CAD build for the part. Positions are in the model's coordinates, mm. A direction names the side the tool comes from. Round coordinates to 2 decimals unless told otherwise and drop trailing zeros. Loops run counter-clockwise (first coordinate to the right, second up) from the corner with the lowest first, then second, coordinate; pieces in that order, holes last. Notation, with made-up numbers: (40.5, 5.5) - (90.5, 5.5) arc R10 cw to (90.5, 9.5) - close; hole circle Ø11 at (50.5, -28.5). An arc over 180 degrees is marked (long way). Use one line per item in the form item = value.
from build123d import *

# Parameters (mm, degrees)
SZKIC2_R                         = 1.65
DODANIE_WYCI_GNI_CIE1_DEPTH      = 3
DODANIE_WYCI_GNI_CIE2_DEPTH      = 5
DODANIE_WYCI_GNI_CIE3_REACH      = 30.62
DODANIE_WYCI_GNI_CIE3_START      = -1
SZKIC7_R                         = 5
SZKIC9_W                         = 12
SZKIC9_H                         = 12
DODANIE_WYCI_GNI_CIE4_DEPTH      = 16
SZKIC10_R                        = 4.1
WYTNIJ_WYCI_GNI_CIE1_DEPTH       = 18
SZKIC12_R                        = 37.17284924
WYTNIJ_WYCI_GNI_CIE2_DEPTH       = 43.690783477
SZKIC13_R                        = 3
WYTNIJ_WYCI_GNI_CIE3_DEPTH       = 42.220824259
SZKIC14_R                        = 1.65
WYTNIJ_WYCI_GNI_CIE4_DEPTH       = 42.220824259
DODANIE_WYCI_GNI_CIE5_DEPTH      = 3
DODANIE_WYCI_GNI_CIE5_DEPTH_BACK = 6
DODANIE_WYCI_GNI_CIE6_REACH      = 55.451
SZKIC16_W                        = 12
SZKIC16_H                        = 5.223766812
SZKIC17_R                        = 1.65
WYTNIJ_WYCI_GNI_CIE5_DEPTH       = 54.450515696
WYTNIJ_WYCI_GNI_CIE6_DEPTH       = 1


with BuildPart() as part:
    # Szkic2 → Dodanie-wyciągnięcie1 (new body)
    with BuildSketch(Plane(origin=(0, 0, 0), x_dir=(1, 0, 0), z_dir=(0, 1, 0))):
        with BuildLine():
            Line((4, 11), (4, -11))
            ThreePointArc((4, -11), (0, -15), (-4, -11))
            Line((-4, -11), (-4, 11))
            ThreePointArc((-4, 11), (0, 15), (4, 11))
        make_face()
        with Locations(Location((0, -11, 0), (0, 0, 270))):
            Circle(SZKIC2_R, mode=Mode.SUBTRACT)
        with Locations(Location((0, 11, 0), (0, 0, 270))):
            Circle(SZKIC2_R, mode=Mode.SUBTRACT)
    extrude(amount=DODANIE_WYCI_GNI_CIE1_DEPTH)

    # Szkic3 → Dodanie-wyciągnięcie2 (add)
    with BuildSketch(Plane(origin=(0, 3, 0), x_dir=(1, 0, 0), z_dir=(0, 1, 0))):
        Polygon((6, 16), (6, -14), (6, -20), (-6, -20), (-6, -14), (-6, 16), (-6, 22), (6, 22), align=None)
        with BuildLine():
            Line((3, 11), (3, -11))
            ThreePointArc((3, -11), (0, -14), (-3, -11))
            Line((-3, -11), (-3, 11))
            ThreePointArc((-3, 11), (0, 14), (3, 11))
        make_face(mode=Mode.SUBTRACT)
    extrude(amount=-DODANIE_WYCI_GNI_CIE2_DEPTH)

    # Dodanie-wyciągnięcie3: up to this face of the body (flat: up to its plane)
    dodanie_wyci_gni_cie3_end = Plane(part.part.faces().sort_by_distance((0, 0, 0))[0])
    # Szkic7 → Dodanie-wyciągnięcie3 (add, up to the picked face)
    with BuildSketch(Plane(origin=(0, -7.995190528, -4.616025404), x_dir=(1, 0, 0), z_dir=(0, -0.866025403784438, -0.500000000000001)).offset(DODANIE_WYCI_GNI_CIE3_START), mode=Mode.PRIVATE) as dodanie_wyci_gni_cie3_sk1:
        with Locations((0, -15.5)):
            Circle(SZKIC7_R)
    dodanie_wyci_gni_cie3_tool1 = split(extrude(dodanie_wyci_gni_cie3_sk1.sketch, amount=-DODANIE_WYCI_GNI_CIE3_REACH, mode=Mode.PRIVATE), bisect_by=dodanie_wyci_gni_cie3_end, keep=Keep.BOTH, mode=Mode.PRIVATE)
    dodanie_wyci_gni_cie3 = dodanie_wyci_gni_cie3_tool1.solids().sort_by(Axis((0, 0.620835, -17.539419), (0, 0.866025403784438, 0.500000000000001)))[0]
    add(dodanie_wyci_gni_cie3)

    # Szkic8 → Wyciągnięcie po profilach1 section 0
    with BuildSketch(Plane(origin=(0, -7.129165125, -4.116025404), x_dir=(-1, 0, 0), z_dir=(0, 0.8660254037844382, 0.5000000000000011))):
        with BuildLine():
            Line((-6, -20.5), (-6, -10.5))
            Line((-6, -10.5), (6, -10.5))
            Line((6, -10.5), (6, -20.5))
            Line((6, -20.5), (-6, -20.5))
        make_face()
    # Szkic5 → Wyciągnięcie po profilach1 section 1
    with BuildSketch(Plane(origin=(0, -12, -12), x_dir=(1, 0, 0), z_dir=(0, 0.7071067811865464, 0.7071067811865488))):
        with BuildLine():
            Line((-6, 18), (-6, 6))
            Line((-6, 6), (6, 6))
            Line((6, 6), (6, 18))
            Line((6, 18), (-6, 18))
        make_face()
    wyci_gni_cie_po_profilach1 = loft()

    # Szkic9 → Dodanie-wyciągnięcie4 (add)
    with BuildSketch(Plane(origin=(0, -12, -12), x_dir=(1, 0, 0), z_dir=(0, -0.7071067811865465, -0.7071067811865487))):
        with Locations((0, -12.018801083)):
            Rectangle(SZKIC9_W, SZKIC9_H)
    dodanie_wyci_gni_cie4 = extrude(amount=DODANIE_WYCI_GNI_CIE4_DEPTH)

    # Szkic10 → Wytnij-wyciągnięcie1 (cut)
    with BuildSketch(Plane(origin=(0, -23.313708499, -23.313708499), x_dir=(1, 0, 0), z_dir=(0, -0.7071067811865465, -0.7071067811865486))):
        with Locations(Location((0, -12, 0), (0, 0, 270))):
            Circle(SZKIC10_R)
    wytnij_wyci_gni_cie1 = extrude(amount=-WYTNIJ_WYCI_GNI_CIE1_DEPTH, mode=Mode.SUBTRACT)

    # Szkic12 → Wytnij-wyciągnięcie2 (cut, through all)
    with BuildSketch(Plane(origin=(0, 3, 0), x_dir=(1, 0, 0), z_dir=(0, 1, 0))):
        Circle(SZKIC12_R)
    wytnij_wyci_gni_cie2 = extrude(amount=WYTNIJ_WYCI_GNI_CIE2_DEPTH, mode=Mode.SUBTRACT)

    # Szkic13 → Wytnij-wyciągnięcie3 (cut, through all)
    with BuildSketch(Plane.XZ):
        with Locations((0, -11)):
            Circle(SZKIC13_R)
    wytnij_wyci_gni_cie3 = extrude(amount=WYTNIJ_WYCI_GNI_CIE3_DEPTH, mode=Mode.SUBTRACT)

    # Lustro1: Dodanie-wyciągnięcie3, Wyciągnięcie po profilach1, Dodanie-wyciągnięcie4, Wytnij-wyciągnięcie1, Wytnij-wyciągnięcie2, Wytnij-wyciągnięcie3 across plane
    add(dodanie_wyci_gni_cie3.mirror(Plane.XY))
    add(wyci_gni_cie_po_profilach1.mirror(Plane.XY))
    add(dodanie_wyci_gni_cie4.mirror(Plane.XY))
    add(wytnij_wyci_gni_cie1.mirror(Plane.XY), mode=Mode.SUBTRACT)
    add(wytnij_wyci_gni_cie2.mirror(Plane.XY), mode=Mode.SUBTRACT)
    add(wytnij_wyci_gni_cie3.mirror(Plane.XY), mode=Mode.SUBTRACT)

    # Szkic14 → Wytnij-wyciągnięcie4 (cut, through all)
    with BuildSketch(Plane.XZ):
        with Locations(Location((0, 11, 0), (0, 0, 90))):
            Circle(SZKIC14_R)
    extrude(amount=-WYTNIJ_WYCI_GNI_CIE4_DEPTH, mode=Mode.SUBTRACT)

    # Szkic15 → Dodanie-wyciągnięcie5 (add, two sides: drawn at the far end of the back side and taken through both)
    with BuildSketch(Plane(origin=(0, 0, 0), x_dir=(0, 0, -1), z_dir=(1, 0, 0)).offset(-DODANIE_WYCI_GNI_CIE5_DEPTH_BACK)):
        Polygon((-25.448323216, -16.936453095), (-6.384776311, -36), (6.384776311, -36), (25.448323216, -16.936453095), (22.619896091, -14.10802597), (4.727922061, -32), (-4.727922061, -32), (-22.619896091, -14.10802597), align=None)
    extrude(amount=DODANIE_WYCI_GNI_CIE5_DEPTH + DODANIE_WYCI_GNI_CIE5_DEPTH_BACK)

    # Szkic16 → Dodanie-wyciągnięcie6 (add, up to next)
    with BuildSketch(Plane(origin=(0, 3, 0), x_dir=(1, 0, 0), z_dir=(0, 1, 0)), mode=Mode.PRIVATE) as dodanie_wyci_gni_cie6_sk1:
        with Locations((0, -19.402002131)):
            Rectangle(SZKIC16_W, SZKIC16_H)
    dodanie_wyci_gni_cie6_tool1 = extrude(dodanie_wyci_gni_cie6_sk1.sketch, amount=-DODANIE_WYCI_GNI_CIE6_REACH, mode=Mode.PRIVATE) - part.part
    add(dodanie_wyci_gni_cie6_tool1.solids().sort_by_distance((0, 3, 19.402002))[0])

    # Szkic17 → Wytnij-wyciągnięcie5 (cut, through all)
    with BuildSketch(Plane(origin=(0, 3, 0), x_dir=(1, 0, 0), z_dir=(0, 1, 0))):
        with Locations(Location((0, 11, 0), (0, 0, 270))):
            Circle(SZKIC17_R)
        with Locations(Location((0, -11, 0), (0, 0, 270))):
            Circle(SZKIC17_R)
    extrude(amount=-WYTNIJ_WYCI_GNI_CIE5_DEPTH, mode=Mode.SUBTRACT)

    # Szkic18 → Wytnij-wyciągnięcie6 (cut)
    with BuildSketch(Plane.ZY.offset(-6)):
        Polygon((29.184280312, -7.406799418), (25.575092277, -7.406799418), (25.575092277, -8.736500273), (27.854579457, -8.736500273), (27.854579457, -10.16117976), (25.575092277, -10.16117976), (25.575092277, -11.490880615), (27.854579457, -11.490880615), (27.854579457, -14.815132751), (29.184280312, -14.815132751), align=None)
    extrude(amount=WYTNIJ_WYCI_GNI_CIE6_DEPTH, mode=Mode.SUBTRACT)


solid = part.part
1) Flat gauge pins, fed straight in: pin 1 (0.8 mm diameter, centred on x = 5.5, z = 28.5, fed in from +Y); pin 2 (4 mm diameter, centred on x = 0, z = 11, fed in from -Y); pin 3 (2.5 mm diameter, centred on x = 0, z = -11, fed in from +Y); pin 4 (6 mm diameter, centred on x = 3.5, y = -8.5, fed in from -Z). Where does each tip first touch, or does it go through?
Report:
pin_1 = -2.62
pin_2 = -33.38
pin_3 = through
pin_4 = -36.05
2) Drill centre lines: probe 1 along X at (y, z) = (-28.5, 11); probe 2 along Y at (x, z) = (-4.5, -3); probe 3 along X at (y, z) = (2, 11). Where is each one in solid material? Low to high.
Report:
probe_1 = -6 to -1.65, 1.65 to 3
probe_2 = -36 to -32, -2 to 3
probe_3 = -6 to -1.65, 1.65 to 6
3) Two-plate mould, pull along Z, no slides. Class faces 1 (the cylindrical face through (0.18, -11.45, 22.63)), 2 (the flat face through (-0.08, -4.84, 30.32)), 3 (the flat face through (-4.08, -13.93, -32.7)): +Z half, -Z half, draft (parallel to the pull), parting line (faces both ways), or undercut.
Report:
face_1 = undercut
face_2 = +Z half
face_3 = -Z half
4) Tool access for faces 4 (the flat face through (-0.08, 1.85, -23.39)), 5 (the flat face through (-1.56, -23.18, 13.55)), 6 (the flat face through (0.06, -2.14, -19.03)): list every direction of +Z, -Z, +X, -X, +Y, -Y with a clear straight run to the whole face (end or side of a thin tool).
Report:
face_4 = -Z, +X, -X, +Y
face_5 = +X, -X
face_6 = none
5) Slice it at A-A (y = -25). Write the cut outline in (x, z).
Report:
outline = (-6, -17.38) - (3, -17.38) - (3, -11.73) - (1.48, -11.73) arc R1.65 cw to (-1.48, -11.73) - (-6, -11.73) - close; (-6, 11.73) - (-1.48, 11.73) arc R1.65 cw to (1.48, 11.73) - (3, 11.73) - (3, 17.38) - (-6, 17.38) - close
6) Slice it at B-B (z = -21). State how many separate pieces and enclosed holes the cut face has, plus the area to 3 significant figures.
Report:
separate_pieces = 2
enclosed_holes = 1
area = 170 mm^2
